Part print with two shaded views. Sizes in mm from the minimum x, y, z corner. A direction names the side the tool comes from. Round coordinates to 2 decimals unless told otherwise and drop trailing zeros. Write each loop counter-clockwise with the first axis right and the second up, starting at its lowest first coordinate (ties: lowest second). Pieces come first, ordered by that corner, then holes.
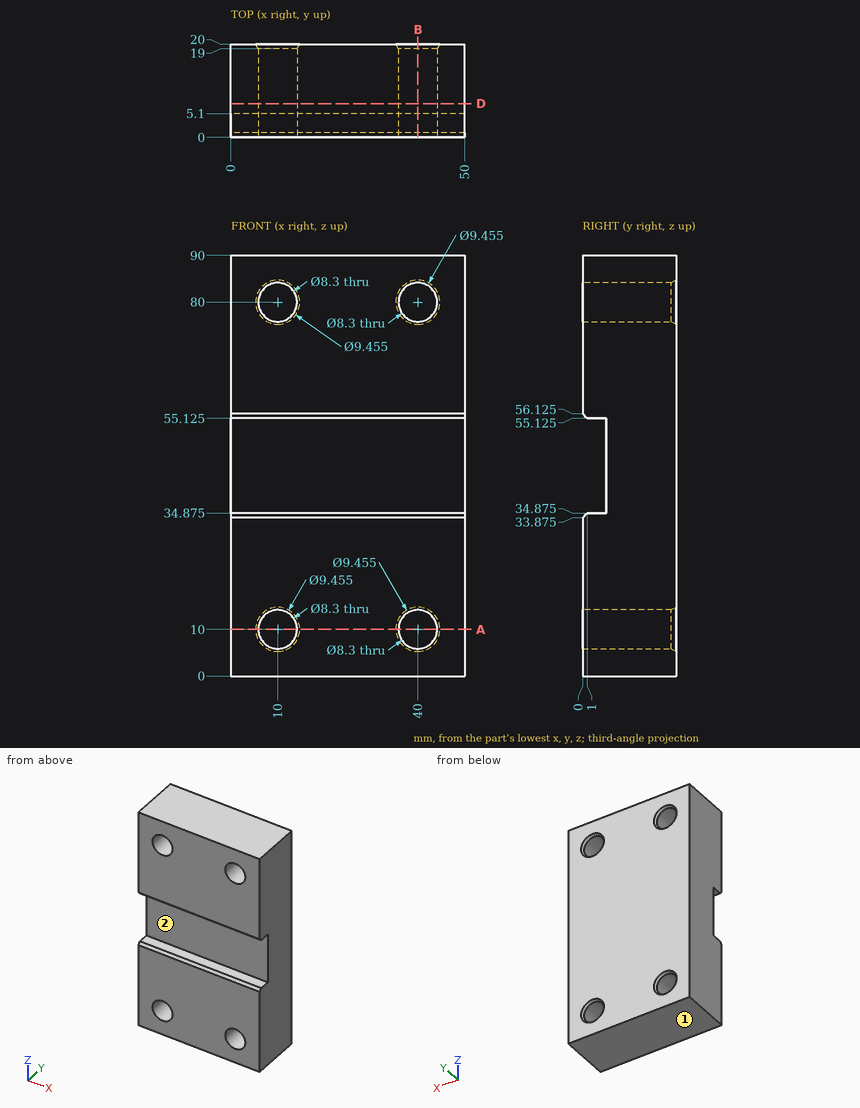
Q1. Cut at A-A on z = 10. Write the cut outline in (x, y).
Values follow:
outline: (0, 0) - (5.85, 0) - (5.85, 19) - (5.27, 20) - (0, 20) - close; (14.15, 0) - (35.85, 0) - (35.85, 19) - (35.27, 20) - (14.73, 20) - (14.15, 19) - close; (44.15, 0) - (50, 0) - (50, 20) - (44.73, 20) - (44.15, 19) - close
Q2. Which spindle directions (+Z, -Z, +X, -X, +Y, -Y) get a long thin tool onto all of the face, cutting with end or side? Do the marked faces 1 and 2. Say none if no direction does.
Values follow:
face 1: -Z, +X, -X, +Y, -Y
face 2: +X, -X, -Y
Q3. Cut at B-B on x = 40. State how many separate pieces and enclosed holes the cut face has, plus the area to 3 significant figures.
Values follow:
separate pieces: 3
enclosed holes: 0
area: 1,360 mm2
Q4. Cut at D-D on y = 7.25. Write the cut outline in (x, z), plus the area to 3 significant figures.
Values follow:
outline: (0, 0) - (50, 0) - (50, 90) - (0, 90) - close; hole circle Ø8.3 at (10, 10); hole circle Ø8.3 at (10, 80); hole circle Ø8.3 at (40, 10); hole circle Ø8.3 at (40, 80)
area: 4,280 mm2
Q5. Drop flat-ended pins along their axis: pin 1 (9.5 mm diameter, centred on x = 10, z = 10, fed in from -Y); pin 2 (4 mm diameter, centred on x = 38, z = 54, fed in from -Y) (1 decimal). Give the stop position or say it passes through.
Values follow:
pin 1: stops at y = 0
pin 2: stops at y = 0.1
Q6. Wall check: L1, parallel to X at y = 9.25, z = 80; L2, parallel to X at y = 13.75, z = 6.5; L3, parallel to Z at x = 37.5, y = 5.5. Give the ranges that are in metal, low to high.
Values follow:
L1: x = 0 to 5.85, 14.15 to 35.85, 44.15 to 50
L2: x = 0 to 7.77, 12.23 to 37.77, 42.23 to 50
L3: z = 0 to 6.69, 13.31 to 76.69, 83.31 to 90
